from build123d import *

# Parameters (mm, degrees)
EXTRUDE_1_DEPTH     = 20
EXTRUDE_2_DEPTH     = 20
CUT_EXTRUDE_1_DEPTH = 15


with BuildPart() as part:
    # 草圖1 → 填料-伸長1 (new body)
    with BuildSketch(Plane(origin=(0, 0, 0), x_dir=(1, 0, 0), z_dir=(0, 1, 0))):
        Polygon((-5, 5), (-5, -10), (15, -5), (15, 5), align=None)
    extrude(amount=EXTRUDE_1_DEPTH)

    # 草圖1<3> → 填料-伸長2 (add)
    with BuildSketch(Plane(origin=(0, 0, 0), x_dir=(1, 0, 0), z_dir=(0, 1, 0))):
        Polygon((-15, -10), (-5, -10), (-5, 5), (15, 5), (15, 10), (-15, 10), align=None)
    extrude(amount=EXTRUDE_2_DEPTH)

    # 草圖2 → 除料-伸長1 (cut)
    with BuildSketch(Plane.XY.offset(10)):
        Polygon((-5, 20), (15, 5), (15, 20), align=None)
    extrude(amount=-CUT_EXTRUDE_1_DEPTH, mode=Mode.SUBTRACT)


solid = part.part
The model under review builds one solid part; all positions refer to its coordinate system, in mm. A direction names the side the tool comes from. Give positions to 0.01 mm unless a question says otherwise; leave off trailing zeros. Order: outer loops, then holes, each group sorted by start corner. A loop starts at its lowest first (then second) coordinate and runs counter-clockwise, first axis right, second up. Notation, with made-up numbers: M 47,51 L 95,51 A19 cw 95,83 Z; hole C 10.5,50 d11. An arc over 180 degrees is marked long. Answer in a Markdown table with one row per item. Add a question column.
1. Add section A-A on y = 4. State the section outline as (x, z) points, plus the area to 3 significant figures.
2. Add section C-C on x = 1. State the section outline as (y, z) points, plus the area to 3 significant figures.
3. To check wall thickness, follow line 1 along Z through (x, y) = (12, 16.25); line 2 along Y through (x, z) = (13, -3.5); line 3 along Z through (x, y) = (-2.75, 6.5). State the ranges of each line that lie inside material, in increasing order.
4. Add section B-B on z = -3.25. State the section outline as (x, y) points.
5. Add section D-D on y = 14.75. State the section outline as (x, z) points.
6. For pin 1 Ø5 at (x, z) = (12, 3) entering from +Y (3 decimals); pin 2 Ø12 at (x, y) = (5, 11.5) entering from +Z; pin 3 Ø4 at (x, y) = (9, 15.5) entering from +Z, all flat-tipped, find the tip position at first contact; note any pin that passes through.
7. Machinability: for faces 1 (the flat face through (0, 0, 0)), 2 (the flat face through (4.86, 12.605, 0.938)), which of the approach directions +Z, -Z, +X, -X, +Y, -Y give a long, thin tool a straight path to every point of the face, cutting with its end or side? Answer none if there is none.
The answers:
| question | item | result |
|---|---|---|
| 1 | outline | M -15,-10 L 15,-10 L 15,5 L -5,10 L -15,10 Z |
| 1 | area | 550 mm2 |
| 2 | outline | M 0,-10 L 20,-10 L 20,-5 L 15.5,-5 L 15.5,8.5 L 0,8.5 Z |
| 2 | area | 309 mm2 |
| 3 | line 1 | -10 to -5 |
| 3 | line 2 | 0 to 6.5 |
| 3 | line 3 | -10 to 9.44 |
| 4 | outline | M -15,0 L 15,0 L 15,5 L -5,20 L -15,20 Z |
| 5 | outline | M -15,-10 L 15,-10 L 15,-5 L 2,-5 L 2,8.25 L -5,10 L -15,10 Z |
| 6 | pin 1 | y = 9.125 |
| 6 | pin 2 | z = 9 |
| 6 | pin 3 | z = -5 |
| 7 | face 1 | +Z, -Z, +X, -X, -Y |
| 7 | face 2 | +Z, +X, +Y |
